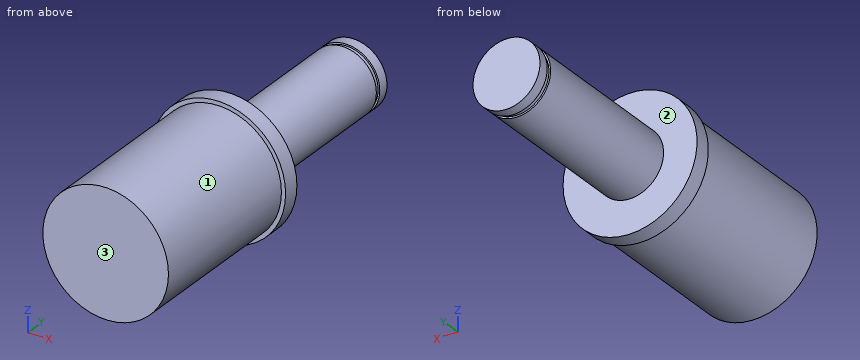
```python
from build123d import *

# Parameters (mm, degrees)
F0_R      = 18.75
F1_DEPTH  = 50
F2_R      = 20
F3_DEPTH  = 5
F5_R      = 10
F6_DEPTH  = 50
F8_R      = 9.5
F9_DEPTH  = 1.5
F11_R     = 10
F12_DEPTH = 3.2


with BuildPart() as f1:
    # F0 (on Front) → F1 (new body)
    with BuildSketch(Plane.XZ):
        Circle(F0_R)
    extrude(amount=F1_DEPTH)

    # F2 (on Front) → F3 (join)
    with BuildSketch(Plane.XZ):
        Circle(F2_R)
    extrude(amount=-F3_DEPTH)

    # F5 (on offset) → F6 (join)
    with BuildSketch(Plane(origin=(0, 5, 0), x_dir=(1, 0, 0), z_dir=(0, 1, 0))):
        Circle(F5_R)
    extrude(amount=F6_DEPTH)

    # F8 (on offset) → F9 (join)
    with BuildSketch(Plane(origin=(0, 55, 0), x_dir=(1, 0, 0), z_dir=(0, 1, 0))):
        Circle(F8_R)
    extrude(amount=F9_DEPTH)

    # F11 (on offset) → F12 (join)
    with BuildSketch(Plane(origin=(0, 56.5, 0), x_dir=(1, 0, 0), z_dir=(0, 1, 0))):
        Circle(F11_R)
    extrude(amount=F12_DEPTH)


solid = f1.part
```
Could you check a few things on this model? Use its own coordinates, in mm. Face numbers are marked on the shaded views. A direction names the side the tool comes from. Round coordinates to 2 decimals unless told otherwise and drop trailing zeros. Write each loop counter-clockwise with the first axis right and the second up, starting at its lowest first coordinate (ties: lowest second). Pieces come first, ordered by that corner, then holes. Notation, with made-up numbers: M 74,-16.5 L 80,-16.5 A29 cw 80,13.5 Z; hole C -38,-35 d6. An arc over 180 degrees is marked long. Answer in a Markdown table with one row per item. Add a question column.
Q1. If I drill on line 1 (Y direction, x = 14.5, z = 0); line 2 (Z direction, x = 0.5, y = -17.5); line 3 (Z direction, x = -0.5, y = 32), over which ranges is the centre line in solid material (lowest first)? Write a range as from..to.
Q2. Imagine slicing it at A-A (z = 0). Please give me the cut outline in (x, y), then the cut area to 3 significant figures.
Q3. Will these pins go through, and if not, where does the flat tip stop? pin 1 Ø8 at (x, y) = (0, 20.5) entering from +Z; pin 2 Ø4 at (x, y) = (2.5, 17) entering from -Z; pin 3 Ø8 at (x, y) = (8, -11.5) entering from +Z.
Q4. Imagine slicing it at D-D (x = 11). Please give me the cut outline in (y, z).
Q5. Imagine slicing it at C-C (y = -8). Please give me the cut outline in (x, z).
Q6. Imagine slicing it at B-B (x = 0). Please give me the cut outline in (y, z).
Q7. On a 3-axis mill with a long thin cutter (end or side, diameter ignored), from which of +Z, -Z, +X, -X, +Y, -Y can I reach the whole of each face in a straight line? I mean the marked faces 1, 2 and 3. Say none if no direction works.
Values:
| question | item | result |
|---|---|---|
| 1 | line 1 | -50..5 |
| 1 | line 2 | -18.74..18.74 |
| 1 | line 3 | -9.99..9.99 |
| 2 | outline | M -20,0 L -18.75,0 L -18.75,-50 L 18.75,-50 L 18.75,0 L 20,0 L 20,5 L 10,5 L 10,55 L 9.5,55 L 9.5,56.5 L 10,56.5 L 10,59.7 L -10,59.7 L -10,56.5 L -9.5,56.5 L -9.5,55 L -10,55 L -10,5 L -20,5 Z |
| 2 | area | 3,170 mm^2 |
| 3 | pin 1 | z = 10 |
| 3 | pin 2 | z = -9.99 |
| 3 | pin 3 | z = 18.32 |
| 4 | outline | M -50,-15.18 L 0,-15.18 L 0,-16.7 L 5,-16.7 L 5,16.7 L 0,16.7 L 0,15.18 L -50,15.18 Z |
| 5 | outline | C 0,0 d37.5 |
| 6 | outline | M -50,-18.75 L 0,-18.75 L 0,-20 L 5,-20 L 5,-10 L 55,-10 L 55,-9.5 L 56.5,-9.5 L 56.5,-10 L 59.7,-10 L 59.7,10 L 56.5,10 L 56.5,9.5 L 55,9.5 L 55,10 L 5,10 L 5,20 L 0,20 L 0,18.75 L -50,18.75 Z |
| 7 | face 1 | -Y |
| 7 | face 2 | +Y |
| 7 | face 3 | +Z, -Z, +X, -X, -Y |
